```python
from build123d import *

# Parameters (mm, degrees)
F0_W     = 25
F0_H     = 20
F0_R     = 4
F1_DEPTH = 25
F2_W     = 15
F2_H     = 10
F3_DEPTH = 1


with BuildPart() as f1:
    # F0 (on Top) → F1 (new body)
    with BuildSketch(Plane.XY):
        Rectangle(F0_W, F0_H)
        Circle(F0_R, mode=Mode.SUBTRACT)
    extrude(amount=F1_DEPTH)

    # F2 (on face) → F3 (cut)
    with BuildSketch(Plane.XY.offset(25)):
        Rectangle(F2_W, F2_H)
    extrude(amount=-F3_DEPTH, mode=Mode.SUBTRACT)


solid = f1.part
```
Can you work these out from the model? Positions are in its coordinate system, mm. A direction names the side the tool comes from. Coordinates: 2 decimals unless noted, no trailing zeros. Loops run counter-clockwise (first coordinate to the right, second up) from the corner with the lowest first, then second, coordinate; pieces in that order, holes last. Notation, with made-up numbers: (-25.5, 89) - (17.5, 89) arc R22 cw to (17.5, 120) - close; hole circle Ø7 at (32, -16.75). An arc over 180 degrees is marked (long way). Answer as CSV lines item,"result". Start each with the question number.
1) Suppose I cut it at B-B (x = 0). Please give me the cut outline in (y, z), plus the area to 3 significant figures.
2) I need wall thicknesses on line 1 (Y direction, x = 0, z = 16.25); line 2 (X direction, y = 0, z = 10.5); line 3 (Z direction, x = -7.25, y = -4.25). Which ranges of each line are inside material? Lowest first, please. Write a range as from..to.
3) Suppose I cut it at A-A (y = 0). Please give me the cut outline in (x, z), plus the area to 3 significant figures.
4) For pin 1 (5 mm diameter, centred on x = 2, y = 2, fed in from +Z); pin 2 (1 mm diameter, centred on x = 5, y = 3, fed in from -Z), each with a flat end and sliding along its axis, tell me the tip position at first contact or that it passes through.
5) Suppose I cut it at D-D (x = -6.5). Please give me the cut outline in (y, z), plus the area to 3 significant figures.
6) Which directions (+Z, -Z, +X, -X, +Y, -Y) give clear straight access to the entire face, cutting with the end or side of a thin tool? Please do faces 1 (the flat face through (7.5, -0.1, 24.5)), 2 (the flat face through (0, 7, 25)).
7) Thinking about a two-plate mould opening in X: for faces 3 (the cylindrical face through (-0.867, -3.905, 11.832)), 4 (the flat face through (0, 10, 12)), 5 (the flat face through (12.5, 0, 12)), 6 (the flat face through (-7.5, -0.1, 24.5)), which applies, pulls with the +X half, pulls with the -X half, needs draft (parallel to the pull), parting line crosses it, or undercut?
8) Suppose I cut it at C-C (z = 3.25). Please give me the cut outline in (x, y).
Check result:
1,outline,"(-10, 0) - (-4, 0) - (-4, 24) - (-5, 24) - (-5, 25) - (-10, 25) - close; (4, 0) - (10, 0) - (10, 25) - (5, 25) - (5, 24) - (4, 24) - close"
1,area,"298 mm²"
2,line 1,"y = -10..-4, 4..10"
2,line 2,"x = -12.5..-4, 4..12.5"
2,line 3,"z = 0..24"
3,outline,"(-12.5, 0) - (-4, 0) - (-4, 24) - (-7.5, 24) - (-7.5, 25) - (-12.5, 25) - close; (4, 0) - (12.5, 0) - (12.5, 25) - (7.5, 25) - (7.5, 24) - (4, 24) - close"
3,area,"418 mm²"
4,pin 1,"stops at z = 24"
4,pin 2,"stops at z = 0"
5,outline,"(-10, 0) - (10, 0) - (10, 25) - (5, 25) - (5, 24) - (-5, 24) - (-5, 25) - (-10, 25) - close"
5,area,"490 mm²"
6,face 1,"+Z"
6,face 2,"+Z, +X, -X, +Y, -Y"
7,face 3,"undercut"
7,face 4,"needs draft"
7,face 5,"pulls with the +X half"
7,face 6,"undercut"
8,outline,"(-12.5, -10) - (12.5, -10) - (12.5, 10) - (-12.5, 10) - close; hole circle Ø8 at (0, 0)"
